from build123d import *

# Parameters (mm, degrees)
F0_W     = 25
F0_H     = 34
F1_DEPTH = 2
F2_W     = 25
F2_H     = 25
F3_DEPTH = 2
F4_R     = 9.75
F5_DEPTH = 2.001
F6_R     = 2


with BuildPart() as f1:
    # F0 (on Front) → F1 (new body)
    with BuildSketch(Plane.XZ):
        with Locations((0, 17)):
            Rectangle(F0_W, F0_H)
    extrude(amount=F1_DEPTH)

    # F2 (on Top) → F3 (join)
    with BuildSketch(Plane.XY):
        with Locations((0, 12.5)):
            Rectangle(F2_W, F2_H)
    extrude(amount=F3_DEPTH)

    # F4 (on face) → F5 (cut, through all)
    with BuildSketch(Plane.XY.offset(2)):
        with Locations((0, 12.5)):
            Circle(F4_R)
    extrude(amount=-F5_DEPTH, mode=Mode.SUBTRACT)

    # F6
    f6_edges = [f1.edges().sort_by_distance(p)[0] for p in [
        (0, -2, 0),
        (0, 0, 2),
    ]]
    fillet(f6_edges, radius=F6_R)


solid = f1.part
Design review of the part built by this model. Coordinates are the model's own, in mm. A direction names the side the tool comes from. Round coordinates to 2 decimals unless told otherwise and drop trailing zeros. Write each loop counter-clockwise with the first axis right and the second up, starting at its lowest first coordinate (ties: lowest second). Pieces come first, ordered by that corner, then holes. Notation, with made-up numbers: (61.5, 2) -> (108.5, 2) arc R16 cw to (108.5, 32) -> close; hole circle Ø5 at (23.25, 37.25). An arc over 180 degrees is marked (long way). One line per item, written item: value. Start each with the question number.
Q1. Tool access review of faces 4 (the face through (-6, 21, 2)), 5 (the face through (-12.5, -1, 9)): name each direction out of +Z, -Z, +X, -X, +Y, -Y from which nothing blocks a thin tool from reaching the whole face with its end or side.
Q2. Add section A-A (x = 0). Give the boundary of the cut face in (y, z).
Q3. Add section C-C (x = -11). Give the boundary of the cut face in (y, z).
Q4. Insertion check: P1, Ø5, axis at x = -9.5, z = 19, coming from the +Y side; P2, Ø12, axis at y = 2, z = 5.5, coming from the -X side. Each pin has a flat end and moves straight along its axis. Give the tip position at first contact, or say it passes through.
Q5. Add section D-D (z = 5). Give the boundary of the cut face in (x, y).
Q6. Add section B-B (y = 12.5). Give the boundary of the cut face in (x, z), then the cut area to 3 significant figures.
Q7. To check wall thickness, follow probe 1 along Z at (x, y) = (11.25, 5.75); probe 2 along Y at (x, z) = (0, 1.25); probe 3 along Y at (x, z) = (8.5, 23). State the ranges of each line that lie inside material, in increasing order.
Q8. The part is to be moulded in two halves that separate along Y. For faces 1 (the face through (0.18, 0.57, 2.6)), 2 (the face through (0, -1, 34)), 3 (the face through (-2.11, 2.98, 1.01)), say which applies: pulls with the +Y half, pulls with the -Y half, needs draft (parallel to the pull), parting line crosses it, or undercut.
Response:
1. face 4: +Z, +X, -X, +Y
1. face 5: +Z, -Z, -X, +Y, -Y
2. outline: (-2, 2) arc R2 ccw to (0, 0) -> (2.75, 0) -> (2.75, 2) -> (2, 2) arc R2 cw to (0, 4) -> (0, 34) -> (-2, 34) -> close; (22.25, 0) -> (25, 0) -> (25, 2) -> (22.25, 2) -> close
3. outline: (-2, 2) arc R2 ccw to (0, 0) -> (25, 0) -> (25, 2) -> (2, 2) arc R2 cw to (0, 4) -> (0, 34) -> (-2, 34) -> close
4. P1: stops at y = 0
4. P2: stops at x = -12.5
5. outline: (-12.5, -2) -> (12.5, -2) -> (12.5, 0) -> (-12.5, 0) -> close
6. outline: (-12.5, 0) -> (-9.75, 0) -> (-9.75, 2) -> (-12.5, 2) -> close; (9.75, 0) -> (12.5, 0) -> (12.5, 2) -> (9.75, 2) -> close
6. area: 11.0 mm^2
7. probe 1: z = 0 to 2
7. probe 2: y = -1.85 to 2.75, 22.25 to 25
7. probe 3: y = -2 to 0
8. face 1: pulls with the +Y half
8. face 2: needs draft
8. face 3: undercut
